```python
from build123d import *

# Parameters (mm, degrees)
F1_DEPTH      = 10.16
F3_DEPTH      = 7.62
F5_DEPTH      = 25.4
F7_DEPTH      = 25.4
F7_DEPTH_BACK = 25.4


with BuildPart() as f1:
    # F0 (on Front) → F1 (new body)
    with BuildSketch(Plane.XZ):
        with BuildLine():
            Line((55.499, 31.877), (-55.499, 31.877))
            ThreePointArc((-55.499, 31.877), (-61.785179, 29.273179), (-64.389, 22.987))
            Line((-64.389, 22.987), (-64.389, -22.987))
            ThreePointArc((-64.389, -22.987), (-61.785179, -29.273179), (-55.499, -31.877))
            Line((-55.499, -31.877), (55.499, -31.877))
            ThreePointArc((55.499, -31.877), (61.785179, -29.273179), (64.389, -22.987))
            Line((64.389, -22.987), (64.389, 22.987))
            ThreePointArc((64.389, 22.987), (61.785179, 29.273179), (55.499, 31.877))
        make_face()
    extrude(amount=F1_DEPTH)

    # F2 (on face) → F3 (cut)
    with BuildSketch(Plane.XZ.offset(10.16)):
        with BuildLine():
            Line((55.499, 29.337), (-55.499, 29.337))
            ThreePointArc((-55.499, 29.337), (-59.989128, 27.477128), (-61.849, 22.987))
            Line((-61.849, 22.987), (-61.849, -22.987))
            ThreePointArc((-61.849, -22.987), (-59.989128, -27.477128), (-55.499, -29.337))
            Line((-55.499, -29.337), (55.499, -29.337))
            ThreePointArc((55.499, -29.337), (59.989128, -27.477128), (61.849, -22.987))
            Line((61.849, -22.987), (61.849, 22.987))
            ThreePointArc((61.849, 22.987), (59.989128, 27.477128), (55.499, 29.337))
        make_face()
    extrude(amount=-F3_DEPTH, mode=Mode.SUBTRACT)

    # F4 (on face) → F5 (cut)
    with BuildSketch(Plane(origin=(0, 0, 0), x_dir=(-1, 0, 0), z_dir=(0, 1, 0))):
        with BuildLine():
            ThreePointArc((-61.394893, -21.146874), (-59.906995, -24.738976), (-56.314893, -26.226874))
            Line((-56.314893, -26.226874), (-56.235034, -26.226874))
            ThreePointArc((-56.235034, -26.226874), (-52.642932, -24.738976), (-51.155034, -21.146874))
            Line((-51.155034, -21.146874), (-51.155034, -12.330383))
            ThreePointArc((-51.155034, -12.330383), (-52.642932, -8.738281), (-56.235034, -7.250383))
            Line((-56.235034, -7.250383), (-56.314893, -7.250383))
            ThreePointArc((-56.314893, -7.250383), (-59.906995, -8.738281), (-61.394893, -12.330383))
            Line((-61.394893, -12.330383), (-61.394893, -21.146874))
        make_face()
    extrude(amount=-F5_DEPTH, mode=Mode.SUBTRACT)

    # F6 (on face) → F7 (cut, two sides)
    with BuildSketch(Plane(origin=(0, 0, 0), x_dir=(-1, 0, 0), z_dir=(0, 1, 0))) as f7_sk:
        Polygon((12.73114, 17.510513), (-32.89561, 0), (12.73114, -17.510513), align=None)
    extrude(amount=F7_DEPTH, mode=Mode.SUBTRACT)
    extrude(f7_sk.sketch, amount=-F7_DEPTH_BACK, mode=Mode.SUBTRACT)


solid = f1.part
```
Input: part model. Units: mm. Frame: model coordinates. A direction names the side the tool comes from. Coordinates: 2 decimals unless noted, no trailing zeros. Loops run counter-clockwise (first coordinate to the right, second up) from the corner with the lowest first, then second, coordinate; pieces in that order, holes last. Notation, with made-up numbers: M -17.5,69 L 5.5,69 A11 ccw 5.5,78 Z; hole C 26,60 d11. An arc over 180 degrees is marked long. Use a Markdown table: item, result. Add a question column.
1) Section D-D, the plane z = -13.5. Return the cut outline in (x, y).
2) Set-up query: faces 4 (the cylindrical face through (-61.72, -5.01, 29.34)), 5 (the cylindrical face through (52.683, -1.252, -24.778)), 6 (the flat face through (61.849, -6, 0)). Return all of +Z, -Z, +X, -X, +Y, -Y with unobstructed straight access to the full face (end or side cutting, diameter ignored); none if empty.
3) Line query: L1, parallel to Z at x = 26, y = -3.5; L2, parallel to X at y = -5.75, z = -6; L3, parallel to Y at x = 2, z = -23.5. Output: solid intervals per line, ascending. Write a range as from..to.
4) Draft query along Z for faces 1 (the flat face through (-15, -10.16, 31)), 2 (the cylindrical face through (59.946, -1.252, -24.699)), 3 (the flat face through (-1, -5, -31.877)). Return one class per face: +Z half, -Z half, draft (parallel to the pull), parting line (faces both ways), or undercut.
5) Section A-A, the plane y = -7.5. Return the cut outline in (x, z), plus the area to 3 significant figures.
6) Section B-B, the plane x = 0.5. Return the cut outline in (y, z), plus the area to 3 significant figures.
7) Section C-C, the plane z = -1.5. Return the cut outline in (x, y).
8) Pin query (flat end, axial travel): P1, Ø4, axis at x = -26, z = -8, coming from the -Y side. Return the tip coordinate at first contact, or that it passes through.
Answer below:
| question | item | result |
|---|---|---|
| 1 | outline | M -64.39,-10.16 L -61.85,-10.16 L -61.85,-2.54 L -12.73,-2.54 L -12.73,0 L -64.39,0 Z; M -2.28,-2.54 L 51.16,-2.54 L 51.16,0 L -2.28,0 Z; M 61.39,-2.54 L 61.85,-2.54 L 61.85,-10.16 L 64.39,-10.16 L 64.39,0 L 61.39,0 Z |
| 2 | face 4 | +Z, -X, +Y, -Y |
| 2 | face 5 | +Y, -Y |
| 2 | face 6 | -Y |
| 3 | L1 | -31.88..-29.34, 29.34..31.88 |
| 3 | L2 | -64.39..-61.85, 61.85..64.39 |
| 3 | L3 | -2.54..0 |
| 4 | face 1 | draft |
| 4 | face 2 | undercut |
| 4 | face 3 | -Z half |
| 5 | outline | M -64.39,-22.99 A8.89 ccw -55.5,-31.88 L 55.5,-31.88 A8.89 ccw 64.39,-22.99 L 64.39,22.99 A8.89 ccw 55.5,31.88 L -55.5,31.88 A8.89 ccw -64.39,22.99 Z; hole M -61.85,-22.99 A6.35 ccw -55.5,-29.34 L 55.5,-29.34 A6.35 ccw 61.85,-22.99 L 61.85,22.99 A6.35 ccw 55.5,29.34 L -55.5,29.34 A6.35 ccw -61.85,22.99 Z |
| 5 | area | 919 mm2 |
| 6 | outline | M -10.16,-31.88 L 0,-31.88 L 0,-12.43 L -2.54,-12.43 L -2.54,-29.34 L -10.16,-29.34 Z; M -10.16,29.34 L -2.54,29.34 L -2.54,12.43 L 0,12.43 L 0,31.88 L -10.16,31.88 Z |
| 6 | area | 137 mm2 |
| 7 | outline | M -64.39,-10.16 L -61.85,-10.16 L -61.85,-2.54 L -12.73,-2.54 L -12.73,0 L -64.39,0 Z; M 28.99,-2.54 L 61.85,-2.54 L 61.85,-10.16 L 64.39,-10.16 L 64.39,0 L 28.99,0 Z |
| 8 | P1 | y = -2.54 |
